Geometry check sheet. Reference: the model listing, model coordinates, mm. A direction names the side the tool comes from. Give positions to 0.01 mm unless a question says otherwise; leave off trailing zeros. Loops run counter-clockwise (first coordinate to the right, second up) from the corner with the lowest first, then second, coordinate; pieces in that order, holes last.
1. Cross-section at C-C, the plane z = -11. Record the cut outline in (x, y), plus the area to 3 significant figures.
2. Release check for a two-part mould opening along Y. For faces 4 (the flat face through (42, 0, -64)), 5 (the cylindrical face through (88.91, 75.13, -64.34)), 6 (the flat face through (63, 152.4, -64)) record: +Y half, -Y half, draft (parallel to the pull), parting line (faces both ways), or undercut.
3. Cross-section at A-A, the plane y = -101.6. Record the cut outline in (x, z).
4. Go/stop test with flat-tipped pins: pin 1 Ø13.5 at (x, z) = (111.5, -62.5) entering from -Y; pin 2 Ø12 at (y, z) = (-51.5, -68) entering from -X; pin 3 Ø5.5 at (x, z) = (96.5, -54.5) entering from +Y; pin 4 Ø15 at (y, z) = (-34.5, -71.5) entering from -X. Record where each tip stops, or that it passes through.
5. Cross-section at B-B, the plane z = -29.5. Record the cut outline in (x, y), plus the area to 3 significant figures.
6. Tool access check on faces 1 (the flat face through (101.6, -114, -107)), 2 (the flat face through (44.45, -26, -64)), 3 (the cylindrical face through (38.09, 77.27, -62.66)). Record the directions out of +Z, -Z, +X, -X, +Y, -Y that give a thin tool (end or side, any length) a straight path to the whole face; none if there is none.
7. Material ranges on L1, parallel to Y at x = 40.5, z = -63; L2, parallel to Y at x = 51, z = -63; L3, parallel to X at y = 22.5, z = -65, recorded low to high.
8. Cross-section at D-D, the plane y = 109.5. Record the cut outline in (x, z).
from build123d import *

# Parameters (mm, degrees)
SKETCH1_W               = 127
SKETCH1_H               = 127
BOSS_EXTRUDE1_DEPTH     = 152.4
SKETCH2_R               = 31.172448383
SKETCH2_R_2             = 38.1
CUT_EXTRUDE1_DEPTH      = 152.4
CUT_EXTRUDE1_DEPTH_BACK = 152.4
SKETCH3_W               = 127
SKETCH3_H               = 127
BOSS_EXTRUDE2_DEPTH     = 152.4
CUT_EXTRUDE_THIN3_DEPTH = 152.4
SKETCH6_R               = 44.45
CUT_EXTRUDE6_DEPTH      = 249.428
CUT_EXTRUDE6_DEPTH_BACK = 249.428
SKETCH7_W               = 25.4
SKETCH7_H               = 101.6
CUT_EXTRUDE8_DEPTH      = 143.256
SKETCH9_R               = 38.1
CUT_EXTRUDE9_DEPTH      = 152.4


with BuildPart() as part:
    # Sketch1 → Boss-Extrude1 (new body)
    with BuildSketch(Plane(origin=(0, 0, 0), x_dir=(1, 0, 0), z_dir=(0, 1, 0))):
        with Locations((63.5, 63.5)):
            Rectangle(SKETCH1_W, SKETCH1_H)
    extrude(amount=BOSS_EXTRUDE1_DEPTH)

    # Sketch2 → Cut-Extrude1 (cut, two sides)
    with BuildSketch(Plane(origin=(0, 0, 0), x_dir=(1, 0, 0), z_dir=(0, 1, 0))) as cut_extrude1_sk:
        with Locations((0, 63.5)):
            Circle(SKETCH2_R)
        with Locations((127, 63.5)):
            Circle(SKETCH2_R_2)
    extrude(amount=CUT_EXTRUDE1_DEPTH, mode=Mode.SUBTRACT)
    extrude(cut_extrude1_sk.sketch, amount=-CUT_EXTRUDE1_DEPTH_BACK, mode=Mode.SUBTRACT)

    # Sketch3 → Boss-Extrude2 (add)
    with BuildSketch(Plane(origin=(0, 0, 0), x_dir=(1, 0, 0), z_dir=(0, 1, 0))):
        with Locations((63.5, 63.5)):
            Rectangle(SKETCH3_W, SKETCH3_H)
    extrude(amount=-BOSS_EXTRUDE2_DEPTH)

    # Sketch5 → Cut-Extrude-Thin3 (cut)
    with BuildSketch(Plane(origin=(0, 0, -129.54), x_dir=(-1, 0, 0), z_dir=(0, 0, -1))):
        Polygon((-127, 0), (-82.55, 0), (-82.55, -50.8), (-127, -50.8), (-127, -48.26), (-85.09, -48.26), (-85.09, -2.54), (-127, -2.54), align=None)
        Polygon((0, -50.8), (-44.45, -50.8), (-44.45, 0), (0, 0), (0, -2.54), (-41.91, -2.54), (-41.91, -48.26), (0, -48.26), align=None)
    extrude(amount=-CUT_EXTRUDE_THIN3_DEPTH, mode=Mode.SUBTRACT)


with BuildPart() as body_2:
    # of the pieces the cut leaves, the one that is kept (cut_extrude_thin3_keep)
    add(part.part.solids().sort_by_distance((0, 152.4, 0))[0])

    # Sketch6 → Cut-Extrude6 (cut, two sides)
    with BuildSketch(Plane(origin=(0, 0, 0), x_dir=(0, 0, -1), z_dir=(1, 0, 0))) as cut_extrude6_sk:
        with Locations(Location((63.5, -101.6, 0), (0, 0, 180))):
            Circle(SKETCH6_R)
    extrude(amount=CUT_EXTRUDE6_DEPTH, mode=Mode.SUBTRACT)
    extrude(cut_extrude6_sk.sketch, amount=-CUT_EXTRUDE6_DEPTH_BACK, mode=Mode.SUBTRACT)

    # Sketch7 → Cut-Extrude8 (cut)
    with BuildSketch(Plane(origin=(0, 0, -129.54), x_dir=(-1, 0, 0), z_dir=(0, 0, -1))):
        with Locations((-114.3, -101.6)):
            Rectangle(SKETCH7_W, SKETCH7_H)
        with Locations((-12.7, -101.6)):
            Rectangle(SKETCH7_W, SKETCH7_H)
    extrude(amount=-CUT_EXTRUDE8_DEPTH, mode=Mode.SUBTRACT)

    # Sketch9 → Cut-Extrude9 (cut)
    with BuildSketch(Plane(origin=(0, 152.4, 0), x_dir=(1, 0, 0), z_dir=(0, 1, 0))):
        with Locations((0, 63.5)):
            Circle(SKETCH9_R)
    extrude(amount=-CUT_EXTRUDE9_DEPTH, mode=Mode.SUBTRACT)


solid = body_2.part
Result:
1. outline: (0, 0) - (44.45, 0) - (44.45, -50.8) - (25.4, -50.8) - (25.4, -152.4) - (101.6, -152.4) - (101.6, -50.8) - (82.55, -50.8) - (82.55, 0) - (127, 0) - (127, 152.4) - (0, 152.4) - close
1. area: 29,000 mm2
2. face 4: undercut
2. face 5: draft
2. face 6: +Y half
3. outline: (25.4, -127) - (101.6, -127) - (101.6, -107.95) - (25.4, -107.95) - close; (25.4, -19.05) - (101.6, -19.05) - (101.6, 0) - (25.4, 0) - close
4. pin 1: passes through
4. pin 2: stops at x = 25.4
4. pin 3: stops at y = -50.8
4. pin 4: stops at x = 44.45
5. outline: (17.19, 0) - (44.45, 0) - (44.45, -50.8) - (25.4, -50.8) - (25.4, -72.97) - (101.6, -72.97) - (101.6, -50.8) - (82.55, -50.8) - (82.55, 0) - (109.81, 0) - (109.81, 152.4) - (17.19, 152.4) - close; (25.4, -152.4) - (101.6, -152.4) - (101.6, -130.23) - (25.4, -130.23) - close
5. area: 19,400 mm2
6. face 1: +Z, -Z, +X, -Y
6. face 2: +Z, -Z, -X
6. face 3: -X, +Y
7. L1: y = -152.4 to -146.05, -57.15 to -50.8, 0 to 152.4
7. L2: y = -152.4 to -146.05, -57.15 to 152.4
7. L3: x = 38.07 to 88.93
8. outline: (0, -127) - (127, -127) - (127, -101.6) arc R38.1 cw to (127, -25.4) - (127, 0) - (0, 0) - (0, -25.4) arc R38.1 cw to (0, -101.6) - close
